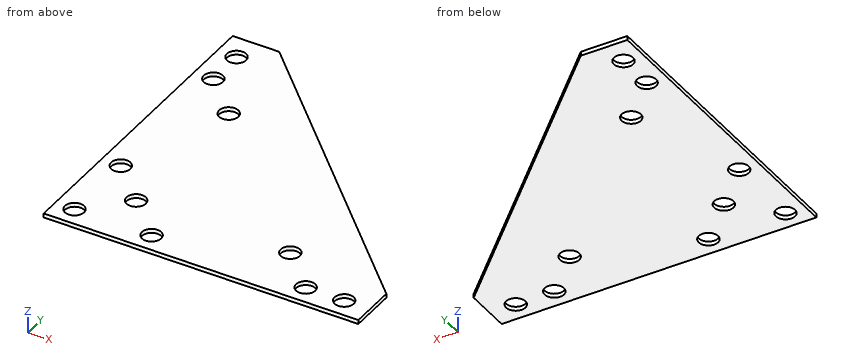
from build123d import *

# Parameters (mm, degrees)
BOSS_EXTRUDE1_DEPTH      = 1.016
BOSS_EXTRUDE1_DEPTH_BACK = 1.016
SKETCH5_R                = 4.7625
CUT_EXTRUDE1_DEPTH       = 2.016
CUT_EXTRUDE1_DEPTH_BACK  = 2.016


with BuildPart() as part:
    # Sketch4 → Boss-Extrude1 (new body, two sides)
    with BuildSketch(Plane.XY) as boss_extrude1_sk:
        Polygon((-54.76875, 77.7875), (-77.7875, 77.7875), (-77.7875, -77.7875), (77.7875, -77.7875), (77.7875, -54.76875), align=None)
    extrude(amount=BOSS_EXTRUDE1_DEPTH)
    extrude(boss_extrude1_sk.sketch, amount=-BOSS_EXTRUDE1_DEPTH_BACK)

    # Sketch5 → Cut-Extrude1 (cut, two sides)
    with BuildSketch(Plane.XY) as cut_extrude1_sk:
        with Locations((-68.2625, 65.0875)):
            Circle(SKETCH5_R)
        with Locations((-68.2625, 46.0375)):
            Circle(SKETCH5_R)
        with Locations((-68.2625, -30.1625)):
            Circle(SKETCH5_R)
        with Locations((-49.2125, 26.9875)):
            Circle(SKETCH5_R)
        with Locations((-49.2125, -49.2125)):
            Circle(SKETCH5_R)
        with Locations((-68.2625, -68.2625)):
            Circle(SKETCH5_R)
        with Locations((-30.1625, -68.2625)):
            Circle(SKETCH5_R)
        with Locations((46.0375, -68.2625)):
            Circle(SKETCH5_R)
        with Locations((26.9875, -49.2125)):
            Circle(SKETCH5_R)
        with Locations((65.0875, -68.2625)):
            Circle(SKETCH5_R)
    extrude(amount=CUT_EXTRUDE1_DEPTH, mode=Mode.SUBTRACT)
    extrude(cut_extrude1_sk.sketch, amount=-CUT_EXTRUDE1_DEPTH_BACK, mode=Mode.SUBTRACT)


solid = part.part
The listing builds one solid part. Answer for the finished solid, in the listing's coordinates (mm). Coordinates: 2 decimals unless noted, no trailing zeros. Loops run counter-clockwise (first coordinate to the right, second up) from the corner with the lowest first, then second, coordinate; pieces in that order, holes last. Notation, with made-up numbers: (56.25, -23.75) -> (101.25, -23.75) arc R18 cw to (101.25, 6.25) -> close; hole circle Ø3 at (3.5, -12). An arc over 180 degrees is marked (long way). Write item = value, one per line. Start each with the question number.
1) A cutting plane is placed at C-C (y = -51). Give the vertices of the cut face in (x, z), then the cut area to 3 significant figures.
2) A cutting plane is placed at A-A (z = 0.65). Count the separate pieces of the cut face and the enclosed holes in it, then the cut area to 3 significant figures.
3) Straight lines are drawn through the part: line 1 (X direction, y = -68.5, z = -0.25); line 2 (X direction, y = -53, z = -0.2); line 3 (X direction, y = -69, z = -0.05). For each, find the intervals that lie inside material, in ascending order. Write a range as from..to.
4) A cutting plane is placed at D-D (x = -46.5). Give the vertices of the cut face in (y, z).
5) A cutting plane is placed at B-B (x = 48). Give the vertices of the cut face in (y, z), then the cut area to 3 significant figures.
Responses:
q1.outline = (-77.79, -1.02) -> (-53.63, -1.02) -> (-53.63, 1.02) -> (-77.79, 1.02) -> close; (-44.8, -1.02) -> (22.57, -1.02) -> (22.57, 1.02) -> (-44.8, 1.02) -> close; (31.4, -1.02) -> (74.02, -1.02) -> (74.02, 1.02) -> (31.4, 1.02) -> close
q1.area = 273 mm²
q2.separate_pieces = 1
q2.enclosed_holes = 10
q2.area = 14,700 mm²
q3.line_1 = -77.79..-73.02, -63.51..-34.92, -25.41..41.28, 50.79..60.33, 69.84..77.79
q3.line_2 = -77.79..-52.1, -46.33..24.1, 29.87..76.02
q3.line_3 = -77.79..-72.97, -63.56..-34.87, -25.46..41.33, 50.74..60.38, 69.79..77.79
q4.outline = (-77.79, -1.02) -> (-53.13, -1.02) -> (-53.13, 1.02) -> (-77.79, 1.02) -> close; (-45.3, -1.02) -> (23.07, -1.02) -> (23.07, 1.02) -> (-45.3, 1.02) -> close; (30.9, -1.02) -> (69.52, -1.02) -> (69.52, 1.02) -> (30.9, 1.02) -> close
q5.outline = (-77.79, -1.02) -> (-72.6, -1.02) -> (-72.6, 1.02) -> (-77.79, 1.02) -> close; (-63.92, -1.02) -> (-24.98, -1.02) -> (-24.98, 1.02) -> (-63.92, 1.02) -> close
q5.area = 89.7 mm²
